Verification items for the finished model (mm, model axes). Give positions to 0.01 mm unless a question says otherwise; leave off trailing zeros. Order: outer loops, then holes, each group sorted by start corner. A loop starts at its lowest first (then second) coordinate and runs counter-clockwise, first axis right, second up. Notation, with made-up numbers: (32, 82) - (75, 82) arc R25 ccw to (75, 96) - close; hole circle Ø6 at (48, -27.75). An arc over 180 degrees is marked (long way). Answer as a JSON object with one key per item and string values. Group by question number.
(1) Depth check by flat-ended pin: pin 1 Ø5 at (x, y) = (148, 33) entering from +Z. Enter the tip coordinate at first touch or a pass-through.
(2) Section check C-C (x = 60). Record the boundary of the cut face in (y, z).
(3) Section check D-D (z = 0.25). Count the separate pieces of the cut face and the enclosed holes in it, then the cut area to 3 significant figures.
(4) Section check A-A (x = -29.5). Record the boundary of the cut face in (y, z), then the cut area to 3 significant figures.
(5) Section check B-B (y = 0). Record the boundary of the cut face in (x, z).
(6) Thickness scan on line 1 (Y direction, x = 60, z = 0.55); line 2 (Y direction, x = 148, z = 0.6); line 3 (Y direction, x = 76, z = 0.65). Record the ranges inside material, lowest first.
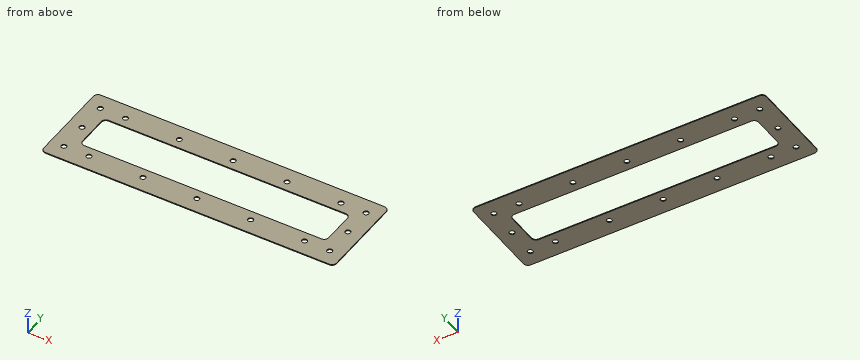
```python
from build123d import *

# Parameters (mm, degrees)
SKETCH1_W            = 326
SKETCH1_H            = 100
SKETCH1_W_2          = 274
SKETCH1_H_2          = 44
BOSS_EXTRUDE1_DEPTH  = 1
FILLET1_R            = 5
M5_CLEARANCE_HOLE1_D = 5.8


with BuildPart() as part:
    # Sketch1 → Boss-Extrude1 (new body)
    with BuildSketch(Plane.XY):
        Rectangle(SKETCH1_W, SKETCH1_H)
        Rectangle(SKETCH1_W_2, SKETCH1_H_2, mode=Mode.SUBTRACT)
    extrude(amount=BOSS_EXTRUDE1_DEPTH)

    # Fillet1
    fillet1_edges = [part.edges().sort_by_distance(p)[0] for p in [
        (-137, 22, 0.5),
        (-137, -22, 0.5),
        (137, -22, 0.5),
        (137, 22, 0.5),
        (163, -50, 0.5),
        (-163, -50, 0.5),
        (-163, 50, 0.5),
        (163, 50, 0.5),
    ]]
    fillet(fillet1_edges, radius=FILLET1_R)

    # M5 Clearance Hole1 (through all)
    with Locations(Plane(origin=(0, 0, 0), x_dir=(-1, 0, 0), z_dir=(0, 0, -1))):
        with Locations((0, 33), (60, 33), (120, 33), (148, 33), (148, 0), (148, -33), (120, -33), (60, -33), (0, -33), (-60, 33), (-60, -33), (-120, -33), (-148, -33), (-148, 0), (-148, 33), (-120, 33)):
            Hole(M5_CLEARANCE_HOLE1_D / 2)


solid = part.part
```
Solutions:
{
 "1": {"pin 1": "passes through"},
 "2": {"outline": "(-50, 0) - (-35.9, 0) - (-35.9, 1) - (-50, 1) - close; (-30.1, 0) - (-22, 0) - (-22, 1) - (-30.1, 1) - close; (22, 0) - (30.1, 0) - (30.1, 1) - (22, 1) - close; (35.9, 0) - (50, 0) - (50, 1) - (35.9, 1) - close"},
 "3": {"separate pieces": "1", "enclosed holes": "17", "area": "20,100 mm2"},
 "4": {"outline": "(-50, 0) - (-22, 0) - (-22, 1) - (-50, 1) - close; (22, 0) - (50, 0) - (50, 1) - (22, 1) - close", "area": "56.0 mm2"},
 "5": {"outline": "(-163, 0) - (-150.9, 0) - (-150.9, 1) - (-163, 1) - close; (-145.1, 0) - (-137, 0) - (-137, 1) - (-145.1, 1) - close; (137, 0) - (145.1, 0) - (145.1, 1) - (137, 1) - close; (150.9, 0) - (163, 0) - (163, 1) - (150.9, 1) - close"},
 "6": {"line 1": "y = -50 to -35.9, -30.1 to -22, 22 to 30.1, 35.9 to 50", "line 2": "y = -50 to -35.9, -30.1 to -2.9, 2.9 to 30.1, 35.9 to 50", "line 3": "y = -50 to -22, 22 to 50"}
}
